from build123d import *

# Parameters (mm, degrees)
SKETCH1_W           = 26
SKETCH1_H           = 18
BOSS_EXTRUDE1_DEPTH = 4
SKETCH2_W           = 3
SKETCH2_H           = 18
BOSS_EXTRUDE2_DEPTH = 41
SKETCH3_R           = 2.75
CUT_EXTRUDE1_DEPTH  = 50.376107583
FILLET1_R           = 3
FILLET2_R           = 5
SKETCH5_R           = 7
BOSS_EXTRUDE3_DEPTH = 2
CUT_EXTRUDE3_REACH  = 49.697
SKETCH7_R           = 2.25
CUT_EXTRUDE4_DEPTH  = 4
CHAMFER1_SIZE       = 2
CUT_EXTRUDE5_DEPTH  = 50.376107601


with BuildPart() as part:
    # Sketch1 → Boss-Extrude1 (new body)
    with BuildSketch(Plane(origin=(0, 0, 0), x_dir=(0, 0, -1), z_dir=(1, 0, 0))):
        Rectangle(SKETCH1_W, SKETCH1_H)
    extrude(amount=BOSS_EXTRUDE1_DEPTH)

    # Sketch2 → Boss-Extrude2 (add)
    with BuildSketch(Plane.ZY):
        with Locations((-11.5, 0)):
            Rectangle(SKETCH2_W, SKETCH2_H)
        with Locations((11.5, 0)):
            Rectangle(SKETCH2_W, SKETCH2_H)
    extrude(amount=BOSS_EXTRUDE2_DEPTH)

    # Sketch3 → Cut-Extrude1 (cut, through all)
    with BuildSketch(Plane.XY.offset(13)):
        with Locations((-35.5, 0)):
            Circle(SKETCH3_R)
    extrude(amount=-CUT_EXTRUDE1_DEPTH, mode=Mode.SUBTRACT)

    # Fillet1
    fillet1_edges = [part.edges().sort_by_distance(p)[0] for p in [
        (4, 0, 13),
        (0, 0, -10),
        (0, 0, 10),
        (4, 0, -13),
    ]]
    fillet(fillet1_edges, radius=FILLET1_R)

    # Fillet2
    fillet2_edges = [part.edges().sort_by_distance(p)[0] for p in [
        (-41, -9, -11.5),
        (-41, 9, -11.5),
        (-41, 9, 11.5),
        (-41, -9, 11.5),
    ]]
    fillet(fillet2_edges, radius=FILLET2_R)

    # Sketch5 → Boss-Extrude3 (add)
    with BuildSketch(Plane.ZY):
        Circle(SKETCH5_R)
    extrude(amount=BOSS_EXTRUDE3_DEPTH)

    # Sketch7 → Cut-Extrude3 (cut, up to next)
    with BuildSketch(Plane(origin=(4, 0, 0), x_dir=(0, 0, -1), z_dir=(1, 0, 0)), mode=Mode.PRIVATE) as cut_extrude3_sk1:
        Circle(SKETCH7_R)
    cut_extrude3_tool1 = extrude(cut_extrude3_sk1.sketch, amount=-CUT_EXTRUDE3_REACH, mode=Mode.PRIVATE) & part.part
    add(cut_extrude3_tool1.solids().sort_by_distance((4, 0, 0))[0], mode=Mode.SUBTRACT)

    # Sketch8 → Cut-Extrude4 (cut)
    with BuildSketch(Plane.ZY.offset(2)):
        Polygon((0, 4.330127019), (-3.75, 2.165063509), (-3.75, -2.165063509), (0, -4.330127019), (3.75, -2.165063509), (3.75, 2.165063509), align=None)
    extrude(amount=-CUT_EXTRUDE4_DEPTH, mode=Mode.SUBTRACT)

    # Chamfer1
    # the kernel refuses this chamfer: 2 mm, written as the material it adds along each edge
    with BuildSketch(Plane(origin=(0, 0, 0), x_dir=(0, 0, 1), z_dir=(0, -1, 0))) as chamfer1_piece_1_section:
        Polygon((7 + CHAMFER1_SIZE, 0), (7, CHAMFER1_SIZE), (7, 0), align=None)
    chamfer1_piece_1 = revolve(axis=Axis((0, 0, 0), (-1, 0, 0)), revolution_arc=180.000000041, mode=Mode.PRIVATE)
    chamfer1_piece_1 = split(chamfer1_piece_1, bisect_by=Plane(origin=(-0.945175713, 9, -3e-09), z_dir=(0, -1, 0)), keep=Keep.TOP, mode=Mode.PRIVATE)
    chamfer1_piece_1 = split(chamfer1_piece_1, bisect_by=Plane(origin=(-2, 8.001744255, -3e-09), z_dir=(1, 0, 0)), keep=Keep.TOP, mode=Mode.PRIVATE)
    add(chamfer1_piece_1)
    with BuildSketch(Plane(origin=(0, 0, 0), x_dir=(0, -7.23525117256177e-10, -1.0), z_dir=(0, 1.0, -7.23525117256177e-10))) as chamfer1_piece_2_section:
        Polygon((7 + CHAMFER1_SIZE, 0), (7, CHAMFER1_SIZE), (7, 0), align=None)
    chamfer1_piece_2 = revolve(axis=Axis((0, 0, 0), (-1, 0, 0)), revolution_arc=179.999999959, mode=Mode.PRIVATE)
    chamfer1_piece_2 = split(chamfer1_piece_2, bisect_by=Plane(origin=(-0.945175715, -9, 3e-09), z_dir=(0, 1, 0)), keep=Keep.TOP, mode=Mode.PRIVATE)
    chamfer1_piece_2 = split(chamfer1_piece_2, bisect_by=Plane(origin=(-2, -8.001744258, 3e-09), z_dir=(1, 0, 0)), keep=Keep.TOP, mode=Mode.PRIVATE)
    add(chamfer1_piece_2)

    # Sketch9 → Cut-Extrude5 (cut, through all)
    with BuildSketch(Plane.XY.offset(13)):
        with BuildLine():
            Line((-19, 6.25), (-10, 6.25))
            ThreePointArc((-10, 6.25), (-3.75, 0), (-10, -6.25))
            Line((-10, -6.25), (-19, -6.25))
            ThreePointArc((-19, -6.25), (-25.25, 0), (-19, 6.25))
        make_face()
    extrude(amount=-CUT_EXTRUDE5_DEPTH, mode=Mode.SUBTRACT)


solid = part.part
The model under review builds one solid part; all positions refer to its coordinate system, in mm. A direction names the side the tool comes from. Round coordinates to 2 decimals unless told otherwise and drop trailing zeros. Loops run counter-clockwise (first coordinate to the right, second up) from the corner with the lowest first, then second, coordinate; pieces in that order, holes last. Notation, with made-up numbers: M -2,61 L 15,61 A22 cw 15,87 Z; hole C 63,-27 d10. An arc over 180 degrees is marked long. Answer as CSV lines item,"result". Start each with the question number.
Item 1: Mouldability with a two-part tool opening along Y and no side actions: class faces 1 (the face through (3.01, 2.23, 0.29)), 2 (the face through (0, -8, 5)), 3 (the face through (-40, 7, -11)), 4 (the face through (-39, -8, -11)) as released by +Y, released by -Y, zero draft, split by the parting line, or undercut.
Item 2: Wall thickness on line 1 (Z direction, x = -26.5, y = 6.75); line 2 (Y direction, x = 2.85, z = 0); line 3 (Y direction, x = -35.5, z = -12.4): over which ranges is each line inside the solid? List them lowest first. Write a range as [from, to].
Item 3: Consider section B-B (x = -35.5). Write out the cut boundary in (y, z), then the cut area to 3 significant figures.
Item 4: Insertion check: P1, Ø5, axis at x = -5.5, z = 6.5, coming from the -Y side; P2, Ø1, axis at y = 6.5, z = -3.5, coming from the -X side; P3, Ø1, axis at y = -8, z = -4.5, coming from the -X side. Each pin has a flat end and moves straight along its axis. Give the tip position at first contact, or say it passes through.
Item 5: Consider section D-D (x = -17.5). Write out the cut boundary in (y, z).
Item 6: For faces 5 (the face through (-26, 0, 10)), 6 (the face through (0, 8, -5)), 7 (the face through (-0.028, 3.232, 1.901)), 8 (the face through (-25.25, -0.14, -11.48)), list the 3-axis set-ups (+Z, -Z, +X, -X, +Y, -Y) from which the entire face can be reached by the end or side of a thin tool; tool diameter is ignored.
Item 7: Consider section A-A (x = -31). Write out the cut boundary in (y, z), then the cut area to 3 significant figures.
Item 8: Consider section C-C (y = 5). State how many separate pieces and enclosed holes the cut face has, then the cut area to 3 significant figures.
Answer:
1,face 1,"undercut"
1,face 2,"zero draft"
1,face 3,"released by +Y"
1,face 4,"released by -Y"
2,line 1,"z = [-13, -10], [10, 13]"
2,line 2,"y = [-9, -2.25], [2.25, 9]"
2,line 3,"y = [-9, -2.75], [2.75, 9]"
3,outline,"M -9,-13 L -2.75,-13 L -2.75,-10 L -9,-10 Z; M -9,10 L -2.75,10 L -2.75,13 L -9,13 Z; M 2.75,-13 L 9,-13 L 9,-10 L 2.75,-10 Z; M 2.75,10 L 9,10 L 9,13 L 2.75,13 Z"
3,area,"75.0 mm^2"
4,P1,"passes through"
4,P2,"stops at x = -2"
4,P3,"stops at x = -0.32"
5,outline,"M -9,-13 L -6.25,-13 L -6.25,-10 L -9,-10 Z; M -9,10 L -6.25,10 L -6.25,13 L -9,13 Z; M 6.25,-13 L 9,-13 L 9,-10 L 6.25,-10 Z; M 6.25,10 L 9,10 L 9,13 L 6.25,13 Z"
6,face 5,"-X, +Y, -Y"
6,face 6,"-X, +Y"
6,face 7,"-X"
6,face 8,"+Z, -Z"
7,outline,"M -9,-13 L 9,-13 L 9,-10 L -9,-10 Z; M -9,10 L 9,10 L 9,13 L -9,13 Z"
7,area,"108 mm^2"
8,separate pieces,"3"
8,enclosed holes,"0"
8,area,"275 mm^2"
